The listing builds one solid part. Answer for the finished solid, in the listing's coordinates (mm). Round coordinates to 2 decimals unless told otherwise and drop trailing zeros. Write each loop counter-clockwise with the first axis right and the second up, starting at its lowest first coordinate (ties: lowest second). Pieces come first, ordered by that corner, then holes. Notation, with made-up numbers: M -25.5,-31 L 26.5,-31 A20 ccw 26.5,-4 Z; hole C 13.5,84.5 d10. An arc over 180 degrees is marked long. Write each question's results on one line, items separated by ' | '.
from build123d import *

# Parameters (mm, degrees)
SKETCH1_W           = 127
SKETCH1_H           = 177.8
BOSS_EXTRUDE1_DEPTH = 3.175
SKETCH3_W           = 63.5
SKETCH3_H           = 63.5
SKETCH3_W_2         = 109.22
SKETCH3_H_2         = 71.12
CUT_EXTRUDE2_DEPTH  = 4.175
BOSS_EXTRUDE2_DEPTH = 3.175
CUT_EXTRUDE3_REACH  = 5.175
SKETCH5_W           = 19.05
SKETCH5_H           = 12.7
SKETCH6_W           = 3.302
SKETCH6_H           = 12.7
CUT_EXTRUDE4_DEPTH  = 4.175
CUT_EXTRUDE5_DEPTH  = 4.175
SKETCH9_W           = 6.477
SKETCH9_H           = 4.064
CUT_EXTRUDE6_DEPTH  = 4.175


with BuildPart() as part:
    # Sketch1 → Boss-Extrude1 (new body)
    with BuildSketch(Plane.XY):
        Rectangle(SKETCH1_W, SKETCH1_H)
    extrude(amount=BOSS_EXTRUDE1_DEPTH)

    # Sketch3 → Cut-Extrude2 (cut, through all)
    with BuildSketch(Plane.XY.offset(3.175)):
        with Locations((0, 44.45)):
            Rectangle(SKETCH3_W, SKETCH3_H)
        with Locations((0, -27.94)):
            Rectangle(SKETCH3_W_2, SKETCH3_H_2)
    extrude(amount=-CUT_EXTRUDE2_DEPTH, mode=Mode.SUBTRACT)

    # Sketch4 → Boss-Extrude2 (add)
    with BuildSketch(Plane.XY.offset(3.175)):
        Polygon((-60.325, 92.075), (-66.675, 92.075), (-66.675, 85.725), (-66.675, 73.025), (-60.325, 73.025), (-60.325, 85.725), (-47.625, 85.725), (-47.625, 92.075), align=None)
        Polygon((60.325, 92.075), (66.675, 92.075), (66.675, 85.725), (66.675, 73.025), (60.325, 73.025), (60.325, 85.725), (47.625, 85.725), (47.625, 92.075), align=None)
    extrude(amount=-BOSS_EXTRUDE2_DEPTH)

    # Sketch5 → Cut-Extrude3 (cut, up to next)
    with BuildSketch(Plane.XY.offset(3.175), mode=Mode.PRIVATE) as cut_extrude3_sk1:
        with Locations((-53.975, -82.55)):
            Rectangle(SKETCH5_W, SKETCH5_H)
    cut_extrude3_tool1 = extrude(cut_extrude3_sk1.sketch, amount=-CUT_EXTRUDE3_REACH, mode=Mode.PRIVATE) & part.part
    add(cut_extrude3_tool1.solids().sort_by_distance((-53.975, -82.55, 3.175))[0], mode=Mode.SUBTRACT)
    # Sketch5 → Cut-Extrude3 (cut, up to next)
    with BuildSketch(Plane.XY.offset(3.175), mode=Mode.PRIVATE) as cut_extrude3_sk2:
        with Locations((53.975, -82.55)):
            Rectangle(SKETCH5_W, SKETCH5_H)
    cut_extrude3_tool2 = extrude(cut_extrude3_sk2.sketch, amount=-CUT_EXTRUDE3_REACH, mode=Mode.PRIVATE) & part.part
    add(cut_extrude3_tool2.solids().sort_by_distance((53.975, -82.55, 3.175))[0], mode=Mode.SUBTRACT)

    # Sketch6 → Cut-Extrude4 (cut, through all)
    with BuildSketch(Plane.XY.offset(3.175)):
        with Locations((-42.799, -82.55)):
            Rectangle(SKETCH6_W, SKETCH6_H)
    extrude(amount=-CUT_EXTRUDE4_DEPTH, mode=Mode.SUBTRACT)

    # Sketch7 → Cut-Extrude5 (cut, through all)
    with BuildSketch(Plane.XY.offset(3.175)):
        Polygon((-41.148, -76.2), (-41.148, -72.136), (44.45, -72.136), (44.45, -76.2), (44.45, -88.9), (-41.148, -88.9), align=None)
    extrude(amount=-CUT_EXTRUDE5_DEPTH, mode=Mode.SUBTRACT)

    # Sketch9 → Cut-Extrude6 (cut, through all)
    with BuildSketch(Plane.XY.offset(3.175)):
        with Locations((-44.3865, -74.168)):
            Rectangle(SKETCH9_W, SKETCH9_H)
        with Locations((47.6885, -74.168)):
            Rectangle(SKETCH9_W, SKETCH9_H)
    extrude(amount=-CUT_EXTRUDE6_DEPTH, mode=Mode.SUBTRACT)


solid = part.part
1) Section C-C (z = 2.3) is taken. Determine the outline of the cut face in (x, y) (3 decimals), then the cut area to 3 significant figures.
Return value:
outline: M -66.675,73.025 L -63.5,73.025 L -63.5,-76.2 L -47.625,-76.2 L -47.625,-72.136 L 50.927,-72.136 L 50.927,-76.2 L 63.5,-76.2 L 63.5,73.025 L 66.675,73.025 L 66.675,92.075 L 47.625,92.075 L 47.625,88.9 L -47.625,88.9 L -47.625,92.075 L -66.675,92.075 Z; hole M -54.61,-63.5 L 54.61,-63.5 L 54.61,7.62 L -54.61,7.62 Z; hole M -31.75,12.7 L 31.75,12.7 L 31.75,76.2 L -31.75,76.2 Z | area: 8,990 mm²
2) Section A-A (y = 36) is taken. Determine the outline of the cut face in (x, z) (3 decimals), then the cut area to 3 significant figures.
Return value:
outline: M -63.5,0 L -31.75,0 L -31.75,3.175 L -63.5,3.175 Z; M 31.75,0 L 63.5,0 L 63.5,3.175 L 31.75,3.175 Z | area: 202 mm²
3) Section B-B (x = 37) is taken. Determine the outline of the cut face in (y, z) (3 decimals).
Return value:
outline: M -72.136,0 L -63.5,0 L -63.5,3.175 L -72.136,3.175 Z; M 7.62,0 L 88.9,0 L 88.9,3.175 L 7.62,3.175 Z
4) Section D-D (x = 6) is taken. Determine the outline of the cut face in (y, z) (3 decimals), then the cut area to 3 significant figures.
Return value:
outline: M -72.136,0 L -63.5,0 L -63.5,3.175 L -72.136,3.175 Z; M 7.62,0 L 12.7,0 L 12.7,3.175 L 7.62,3.175 Z; M 76.2,0 L 88.9,0 L 88.9,3.175 L 76.2,3.175 Z | area: 83.9 mm²
5) Find the intervals of material crossed by line 1 (Y direction, x = -30.5, z = 2.8); line 2 (Y direction, x = -49.5, z = 0.4) (3 decimals); line 3 (Y direction, x = -35.5, z = 1.4), in increasing order.
Return value:
line 1: -72.14 to -63.5, 7.62 to 12.7, 76.2 to 88.9 | line 2: -76.2 to -63.5, 7.62 to 92.075 | line 3: -72.14 to -63.5, 7.62 to 88.9
6) Each of these flat-tipped pins is pushed along its axis until it touches: pin 1 (1.6 mm diameter, centred on y = 53.5, z = 1, fed in from +X); pin 2 (1.6 mm diameter, centred on x = 13.5, z = 1, fed in from +Y); pin 3 (1.6 mm diameter, centred on x = 65.5, z = 2, fed in from -Y) (3 decimals). Where does it stop, or does it pass through?
Return value:
pin 1: x = 63.5 | pin 2: y = 88.9 | pin 3: y = 73.025
